```python
from build123d import *

# Parameters (mm, degrees)
F1_DEPTH = 10
F2_DEPTH = 3
F3_D     = 5
F3_DEPTH = 12
F3_TIP   = 1.5021515476


with BuildPart() as f1:
    # F0 (on Front) → F1 (new body)
    with BuildSketch(Plane.XZ):
        Polygon((0, 19.8648640182), (-15, 0), (-15, -10), (-12, -10), (-12, -1.0054318503), (0, 14.8864593642), (12, -1.0054318503), (12, -10), (15, -10), (15, 0), align=None)
    extrude(amount=F1_DEPTH)

    # F0 (on Front) + F1_face (on face) → F2 (join)
    with BuildSketch(Plane.XZ):
        Polygon((-12, -1.0054318503), (-12, -10), (12, -10), (12, -1.0054318503), (0, 14.8864593642), align=None)
    with BuildSketch(Plane(origin=(0, -10, 4.4015692683), x_dir=(1, 0, 0), z_dir=(0, -1, 0))):
        Polygon((0, 15.4632947499), (-15, -4.4015692683), (-15, -14.4015692683), (-12, -14.4015692683), (-12, -5.4070011186), (0, 10.484890096), (12, -5.4070011186), (12, -14.4015692683), (15, -14.4015692683), (15, -4.4015692683), align=None)
    extrude(amount=F2_DEPTH)

    # F3
    with Locations(Plane(origin=(0, 0, 0), x_dir=(1, 0, 0), z_dir=(0, 1, 0))):
        with Locations((0, 1.5340909595)):
            Hole(F3_D / 2, depth=F3_DEPTH)
            with Locations((0, 0, -(F3_DEPTH + F3_TIP / 2))):  # 118° drill point
                Cone(0, F3_D / 2, F3_TIP, mode=Mode.SUBTRACT)


solid = f1.part
```
Geometry: final body of the model. Coordinates: model frame, mm. A direction names the side the tool comes from. Give positions to 0.01 mm unless a question says otherwise; leave off trailing zeros. Write each loop counter-clockwise with the first axis right and the second up, starting at its lowest first coordinate (ties: lowest second). Pieces come first, ordered by that corner, then holes.
1. Line query: probe 1 along X at (y, z) = (-7.5, -5); probe 2 along X at (y, z) = (-11.5, 9.5); probe 3 along Y at (x, z) = (-5, 5.75). Output: solid intervals per line, ascending.
2. Draft query along X for faces 3 (the flat face through (-15, -6, -5)), 4 (the flat face through (0, -2, -10)), 5 (the flat face through (-12, -8, -6)). Return one class per face: released by +X, released by -X, zero draft, split by the parting line, or undercut.
3. Section query C-C, the plane x = -0.5. Return loops of the section in (y, z), then the cut area to 3 significant figures.
4. Pin query (flat end, axial travel): P1, Ø1, axis at x = 12, z = 7, coming from the -Y side; P2, Ø2, axis at x = 5, y = -5.5, coming from the +Z side. Return the tip coordinate at first contact, or that it passes through.
5. Section query A-A, the plane y = -5.75. Return loops of the section in (x, z).
6. Section query B-B, the plane z = -5.5. Return loops of the section in (x, y).
7. Reachability of faces 1 (the flat face through (-3, -3, 0)), 2 (the flat face through (0, 0, 2)) from +Z, -Z, +X, -X, +Y, -Y: full face, straight path, thin tool, end or side. Return the list, or none.
8. Section query D-D, the plane x = -9. Return loops of the section in (y, z).
Computed:
1. probe 1: x = -15 to -12, 12 to 15
1. probe 2: x = -7.83 to -4.07, 4.07 to 7.83
1. probe 3: y = -3 to 0
2. face 3: released by -X
2. face 4: zero draft
2. face 5: undercut
3. outline: (-13, 14.22) - (-3, 14.22) - (-3, 0.92) - (0, 0.92) - (0, 19.2) - (-13, 19.2) - close; (-3, -10) - (0, -10) - (0, -3.98) - (-3, -3.98) - close
3. area: 123 mm2
4. P1: passes through
4. P2: stops at z = 14.57
5. outline: (-15, -10) - (-12, -10) - (-12, -1.01) - (0, 14.89) - (12, -1.01) - (12, -10) - (15, -10) - (15, 0) - (0, 19.86) - (-15, 0) - close
6. outline: (-15, -13) - (-12, -13) - (-12, -3) - (12, -3) - (12, -13) - (15, -13) - (15, 0) - (-15, 0) - close
7. face 1: -Z, -Y
7. face 2: +Z, -Z, +X, -X, +Y
8. outline: (-13, 2.97) - (-3, 2.97) - (-3, -10) - (0, -10) - (0, 7.95) - (-13, 7.95) - close
